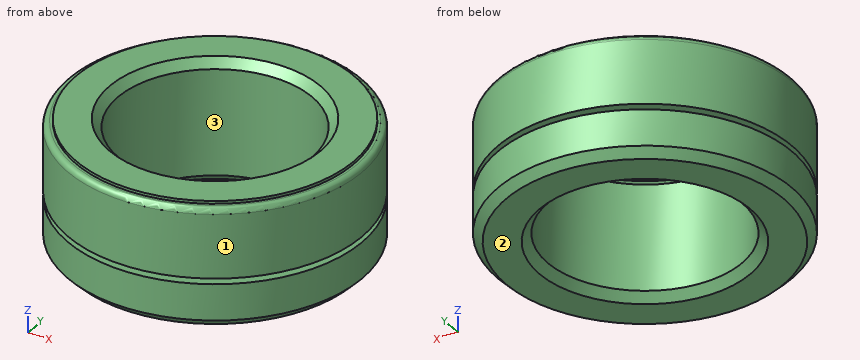
from build123d import *

# Parameters (mm, degrees)
F2_R    = 1
F3_SIZE = 1.5


with BuildPart() as f1:
    # F0 (on Front) → F1 (revolve)
    with BuildSketch(Plane.XZ):
        Polygon((17.5, 22), (17.5, 0), (26.5, 0), (26.5, 8), (21.5, 8), (21.5, 9), (26.5, 9), (26.5, 21.5), (25, 21.5), (25, 22), align=None)
    revolve(axis=Axis((0, 0, 2.07143), (0, 0, 1)))

    # F2
    f2_edges = [f1.edges().sort_by_distance(p)[0] for p in [
        (-26.5, 0, 21.5),
    ]]
    fillet(f2_edges, radius=F2_R)

    # F3
    f3_edges = [f1.edges().sort_by_distance(p)[0] for p in [
        (-26.5, 0, 0),
        (-17.5, 0, 22),
        (-17.5, 0, 0),
    ]]
    chamfer(f3_edges, length=F3_SIZE)


solid = f1.part
Can you work these out from the model? Positions are in its coordinate system, mm. Face numbers are marked on the shaded views. Give positions to 0.01 mm unless a question says otherwise; leave off trailing zeros. Loops run counter-clockwise (first coordinate to the right, second up) from the corner with the lowest first, then second, coordinate; pieces in that order, holes last. Notation, with made-up numbers: M 27.25,67 L 48.25,67 A31 cw 48.25,93 Z; hole C -6.75,72 d4. An arc over 180 degrees is marked long. One line per item, written item: value. Start each with the question number.
1) If I drill on line 1 (Z direction, x = -19.5, y = 10); line 2 (Y direction, x = 0, z = 11); line 3 (X direction, y = 0.5, z = 5), over which ranges is the centre line in solid material (lowest first)? Write a range as [from, to].
2) I'm going to push flat-ended pins straight in: pin 1 (3 mm diameter, centred on y = -4.5, z = 9, fed in from -X); pin 2 (12 mm diameter, centred on x = -20, z = 8, fed in from -Y); pin 3 (10 mm diameter, centred on x = -5, z = 10, fed in from -Y). Where does each tip first touch, or does it pass through?
3) If we section it at A-A, the plane x = 0: Write out the boundary of the cut face in (y, z).
4) If we section it at C-C, the plane z = 18.5: Write out the boundary of the cut face in (x, y).
5) Thinking about a two-plate mould opening in Y: for the marked faces 1, 2 and 3, which applies, +Y half, -Y half, draft (parallel to the pull), parting line (faces both ways), or undercut?
Completed:
1. line 1: z = [0, 8], [9, 22]
1. line 2: y = [-26.5, -17.5], [17.5, 26.5]
1. line 3: x = [-26.5, -17.49], [17.49, 26.5]
2. pin 1: stops at x = -26.33
2. pin 2: stops at y = -22.5
2. pin 3: stops at y = -26.5
3. outline: M -26.5,1.5 L -25,0 L -19,0 L -17.5,1.5 L -17.5,20.5 L -19,22 L -25,22 L -25,21.5 L -25.5,21.5 A1 ccw -26.5,20.5 L -26.5,9 L -21.5,9 L -21.5,8 L -26.5,8 Z; M 17.5,1.5 L 19,0 L 25,0 L 26.5,1.5 L 26.5,8 L 21.5,8 L 21.5,9 L 26.5,9 L 26.5,20.5 A1 ccw 25.5,21.5 L 25,21.5 L 25,22 L 19,22 L 17.5,20.5 Z
4. outline: C 0,0 d53; hole C 0,0 d35
5. face 1: parting line
5. face 2: draft
5. face 3: undercut
